from build123d import *

# Parameters (mm, degrees)
SKETCH1_W               = 15
SKETCH1_H               = 15
SKETCH1_W_2             = 11
SKETCH1_H_2             = 11
BOSS_EXTRUDE1_DEPTH     = 60
CUT_EXTRUDE1_DEPTH      = 63.299678972
CUT_EXTRUDE1_DEPTH_BACK = 63.299678972
SKETCH2_R               = 2


with BuildPart() as part:
    # Sketch1 → Boss-Extrude1 (new, symmetric)
    with BuildSketch(Plane.XY):
        Rectangle(SKETCH1_W, SKETCH1_H)
        Rectangle(SKETCH1_W_2, SKETCH1_H_2, mode=Mode.SUBTRACT)
    extrude(amount=BOSS_EXTRUDE1_DEPTH, both=True)

    # Sketch2 → Cut-Extrude1 (cut, two sides: drawn at the far end of the back side and taken through both)
    with BuildSketch(Plane(origin=(7.5, 0, 0), x_dir=(0, 0, -1), z_dir=(1, 0, 0)).offset(-CUT_EXTRUDE1_DEPTH_BACK)):
        with Locations((-44.599061213, -0.2)):
            Circle(SKETCH2_R)
        with Locations((49, -0.2)):
            Circle(SKETCH2_R)
    extrude(amount=CUT_EXTRUDE1_DEPTH + CUT_EXTRUDE1_DEPTH_BACK, mode=Mode.SUBTRACT)


solid = part.part
For this review, take the finished solid that the model builds, in its own axes (mm). A direction names the side the tool comes from. Give positions to 0.01 mm unless a question says otherwise; leave off trailing zeros. Loops run counter-clockwise (first coordinate to the right, second up) from the corner with the lowest first, then second, coordinate; pieces in that order, holes last. Notation, with made-up numbers: M -9,-7 L 45,-7 A23 ccw 45,27 Z; hole C 65.25,59 d1. An arc over 180 degrees is marked long. Put each result on its own line as item: value. Start each with the question number.
(1) Add section A-A, the plane y = -0.2. Write out the cut boundary in (x, z).
(2) Add section B-B, the plane x = -3.5. Write out the cut boundary in (y, z), then the cut area to 3 significant figures.
(3) Add section C-C, the plane z = -49. Write out the cut boundary in (x, y), then the cut area to 3 significant figures.
(4) Machinability: for faces 1 (the flat face through (-7, 0, -60)), 2 (the flat face through (0, -5.5, 1)), which of the approach directions +Z, -Z, +X, -X, +Y, -Y give a long, thin tool a straight path to every point of the face, cutting with its end or side? Answer none if there is none.
(5) For pin 1 (6 mm diameter, centred on x = 2, y = 0, fed in from +Z), flat-tipped, find the tip position at first contact; note if it passes through.
(6) Wall thickness on L1, parallel to Z at x = 6.05, y = -0.2; L2, parallel to X at y = -0.25, z = 13.5; L3, parallel to Y at x = 6.45, z = -49: over which ranges is each line inside the solid? List them lowest first.
(7) Add section D-D, the plane z = 35.5. Write out the cut boundary in (x, y), then the cut area to 3 significant figures.
(8) The part is to be moulded in two halves that separate along X. For faces 3 (the flat face through (0, -7.5, 1)), 4 (the flat face through (5.5, 0, 1)), 5 (the flat face through (-7.5, 0, 1)), 6 (the flat face through (0, 5.5, 1)), say which applies: +X half, -X half, draft (parallel to the pull), parting line (faces both ways), or undercut.
Result:
1. outline: M -7.5,-60 L -5.5,-60 L -5.5,-51 L -7.5,-51 Z; M -7.5,-47 L -5.5,-47 L -5.5,42.6 L -7.5,42.6 Z; M -7.5,46.6 L -5.5,46.6 L -5.5,60 L -7.5,60 Z; M 5.5,-60 L 7.5,-60 L 7.5,-51 L 5.5,-51 Z; M 5.5,-47 L 7.5,-47 L 7.5,42.6 L 5.5,42.6 Z; M 5.5,46.6 L 7.5,46.6 L 7.5,60 L 5.5,60 Z
2. outline: M -7.5,-60 L -5.5,-60 L -5.5,60 L -7.5,60 Z; M 5.5,-60 L 7.5,-60 L 7.5,60 L 5.5,60 Z
2. area: 480 mm^2
3. outline: M -7.5,-7.5 L 7.5,-7.5 L 7.5,-2.2 L 5.5,-2.2 L 5.5,-5.5 L -5.5,-5.5 L -5.5,-2.2 L -7.5,-2.2 Z; M -7.5,1.8 L -5.5,1.8 L -5.5,5.5 L 5.5,5.5 L 5.5,1.8 L 7.5,1.8 L 7.5,7.5 L -7.5,7.5 Z
3. area: 88.0 mm^2
4. face 1: -Z, +X, -X, +Y, -Y
4. face 2: +Z, -Z
5. pin 1: passes through
6. L1: z = -60 to -51, -47 to 42.6, 46.6 to 60
6. L2: x = -7.5 to -5.5, 5.5 to 7.5
6. L3: y = -7.5 to -2.2, 1.8 to 7.5
7. outline: M -7.5,-7.5 L 7.5,-7.5 L 7.5,7.5 L -7.5,7.5 Z; hole M -5.5,-5.5 L 5.5,-5.5 L 5.5,5.5 L -5.5,5.5 Z
7. area: 104 mm^2
8. face 3: draft
8. face 4: undercut
8. face 5: -X half
8. face 6: undercut
